```python
from build123d import *

# Parameters (mm, degrees)
F3_DEPTH = 10


with BuildPart() as f1:
    # F0 (on Top) → F1 (revolve)
    with BuildSketch(Plane.XY):
        with BuildLine():
            Line((97.4973875252, -38.8161949813), (121.4477377606, -38.8161949813))
            ThreePointArc((121.4477377606, -38.8161949813), (120.5697284263, -19.6675259883), (117.0955747366, -0.8161949813))
            Line((117.0955747366, -0.8161949813), (97.4973875252, -0.8161949813))
            Line((97.4973875252, -0.8161949813), (97.4973875252, -38.8161949813))
        make_face()
        with BuildLine():
            ThreePointArc((117.0955747366, -0.8161949813), (120.5697284263, -19.6675259883), (121.4477377606, -38.8161949813))
            ThreePointArc((121.4477377606, -38.8161949813), (125.914331396, -20.045726455), (127.4973875252, -0.8161949813))
            Line((127.4973875252, -0.8161949813), (117.0955747366, -0.8161949813))
        make_face()
    revolve(axis=Axis((0, 9.7614582628, 0), (0, -1, 0)))

    # F2 (on face) → F3 (cut)
    with BuildSketch(Plane(origin=(0, -0.8161949813, 0), x_dir=(-1, 0, 0), z_dir=(0, 1, 0))):
        with BuildLine():
            Line((-4.9983559861, -97.3691789617), (0.6029718567, -103.4572258853))
            Line((0.6029718567, -103.4572258853), (4.8713640334, -97.375614949))
            ThreePointArc((4.8713640334, -97.375614949), (2.4364429045, -97.4669396268), (0, -97.4973875252))
            ThreePointArc((0, -97.4973875252), (-2.5, -97.465330114), (-4.9983559861, -97.3691789617))
        make_face()
    extrude(amount=-F3_DEPTH, mode=Mode.SUBTRACT)


solid = f1.part
```
Geometry: final body of the model. Coordinates: model frame, mm. A direction names the side the tool comes from. Round coordinates to 2 decimals unless told otherwise and drop trailing zeros. Order: outer loops, then holes, each group sorted by start corner. A loop starts at its lowest first (then second) coordinate and runs counter-clockwise, first axis right, second up. Notation, with made-up numbers: (39, 41) -> (43, 41) arc R13 cw to (43, 47) -> close; hole circle Ø10 at (-20, 52.5). An arc over 180 degrees is marked (long way). Use one line per item in the form item = value.
(1) Section B-B on x = -59.5. Return loops of the section in (y, z).
Results list:
outline = (-38.82, -105.87) arc R112.77 ccw to (-0.82, -112.76) -> (-0.82, -77.24) -> (-38.82, -77.24) -> close; (-38.82, 77.24) -> (-0.82, 77.24) -> (-0.82, 112.76) arc R112.77 ccw to (-38.82, 105.87) -> close
(2) Section A-A on z = 0. Return loops of the section in (x, y).
Results list:
outline = (-127.5, -0.82) arc R127.5 ccw to (-121.45, -38.82) -> (-97.5, -38.82) -> (-97.5, -0.82) -> close; (97.5, -38.82) -> (121.45, -38.82) arc R127.5 ccw to (127.5, -0.82) -> (97.5, -0.82) -> close
(3) Draft query along X for faces 1 (the face through (-12.69, -20.08, 96.67)), 2 (the face through (1, -38.816, 100)). Return one class per face: pulls with the +X half, pulls with the -X half, needs draft (parallel to the pull), parting line crosses it, or undercut.
Results list:
face_1 = undercut
face_2 = needs draft
(4) First-contact query: pin 1 Ø3 at (y, z) = (-34, -4) entering from +X; pin 2 Ø1 at (x, y) = (38, -15.5) entering from +Z; pin 3 Ø3 at (x, y) = (-64.5, -29) entering from -Z. Flat tips, straight axial feed; report the tip coordinate or a pass-through.
Results list:
pin_1 = 123.23
pin_2 = 120.88
pin_3 = -107.07
(5) Access query for faces 3 (the face through (-29, -0.816, -94)), 4 (the face through (-2.707, -5.746, -100.459)). Directions: +Z, -Z, +X, -X, +Y, -Y. A direction counts if a zero-diameter tool reaches every point of the face in a straight line with its end or side. Return the directions, or none.
Results list:
face_3 = +Z, -Z, +X, -X, +Y
face_4 = +Y
(6) Ray query, probe 1 along X at (y, z) = (-8.5, 0); probe 2 along X at (y, z) = (-14, 0); probe 3 along Z at (x, y) = (51, -24.5). Return the intervals inside material, ascending. Write a range as [from, to].
Results list:
probe_1 = [-127.22, -97.5], [97.5, 127.22]
probe_2 = [-126.73, -97.5], [97.5, 126.73]
probe_3 = [-114.26, -83.09], [83.09, 114.26]
(7) Section C-C on z = -100.5. Return loops of the section in (x, y).
Results list:
outline = (-78.46, -0.82) arc R78.46 ccw to (-68.19, -38.82) -> (68.19, -38.82) arc R78.46 ccw to (78.46, -0.82) -> (2.12, -0.82) -> (2.12, -10.82) -> (-2.68, -10.82) -> (-2.68, -0.82) -> close
(8) Section D-D on y = -15. Return loops of the section in (x, z), and give its area (3 significant figures).
Results list:
outline = circle Ø253.23 at (0, 0); hole circle Ø194.99 at (0, 0)
area = 20,500 mm^2
